Read the model definition and answer for the solid it produces. Units are mm, in the model's axes. Give positions to 0.01 mm unless a question says otherwise; leave off trailing zeros. Order: outer loops, then holes, each group sorted by start corner. A loop starts at its lowest first (then second) coordinate and runs counter-clockwise, first axis right, second up. Notation, with made-up numbers: (-32.75, -18.5) - (19.25, -18.5) arc R18 ccw to (19.25, 15.5) - close; hole circle Ø2 at (-29.75, 6.25). An arc over 180 degrees is marked (long way). Return JSON: item names as keys, results as strings.
```python
from build123d import *

# Parameters (mm, degrees)
SKETCH_1_W               = 40
SKETCH_1_H               = 20
EXTRUDE_2_DEPTH          = 150
SKETCH_5_R               = 20
EXTRUDE_3_DEPTH          = 20
CUT_EXTRUDE_1_DEPTH      = 153.643375225
CUT_EXTRUDE_1_DEPTH_BACK = 153.643375225
SKETCH_6_R               = 10


with BuildPart() as part:
    # 스케치1 → 보스-돌출2 (new body)
    with BuildSketch(Plane.XY):
        Rectangle(SKETCH_1_W, SKETCH_1_H)
    extrude(amount=EXTRUDE_2_DEPTH)

    # 스케치5 → 보스-돌출3 (add)
    with BuildSketch(Plane(origin=(0, 10, 0), x_dir=(1, 0, 0), z_dir=(0, 1, 0))):
        Circle(SKETCH_5_R)
    extrude(amount=-EXTRUDE_3_DEPTH)

    # 스케치6 → 컷-돌출1 (cut, two sides: drawn at the far end of the back side and taken through both)
    with BuildSketch(Plane(origin=(0, 10, 0), x_dir=(1, 0, 0), z_dir=(0, 1, 0)).offset(-CUT_EXTRUDE_1_DEPTH_BACK)):
        with Locations(Location((0, 0, 0), (0, 0, 180))):
            Circle(SKETCH_6_R)
    extrude(amount=CUT_EXTRUDE_1_DEPTH + CUT_EXTRUDE_1_DEPTH_BACK, mode=Mode.SUBTRACT)


solid = part.part
```
Q1. Determine the mould class of faces 1 (the flat face through (-20, 0, 74)), 2 (the cylindrical face through (10, 0, 0)), 3 (the flat face through (20, 0, 74)) for opening direction X: released by +X, released by -X, zero draft, split by the parting line, or undercut.
Values:
{"face 1": "released by -X", "face 2": "undercut", "face 3": "released by +X"}
Q2. A cutting plane is placed at D-D (x = 12). Write down the section's boundary in (y, z).
Values:
{"outline": "(-10, -16) - (10, -16) - (10, 150) - (-10, 150) - close"}
Q3. Consider L1, parallel to Z at x = 0, y = 2.75; L2, parallel to X at y = 3.5, z = 0; L3, parallel to Z at x = -8.5, y = 8.25. Determine where each line is inside the solid, lowest interval first.
Values:
{"L1": "z = -20 to -10, 10 to 150", "L2": "x = -20 to -10, 10 to 20", "L3": "z = -18.1 to -5.27, 5.27 to 150"}
Q4. A cutting plane is placed at C-C (y = 2.25). Write down the section's boundary in (x, z), and give its area (3 significant figures).
Values:
{"outline": "(-20, 0) arc R20 ccw to (20, 0) - (20, 150) - (-20, 150) - close; hole circle Ø20 at (0, 0)", "area": "6,310 mm²"}
Q5. A cutting plane is placed at A-A (x = 0). Write down the section's boundary in (y, z).
Values:
{"outline": "(-10, -20) - (10, -20) - (10, -10) - (-10, -10) - close; (-10, 10) - (10, 10) - (10, 150) - (-10, 150) - close"}
Q6. A cutting plane is placed at B-B (z = -6.5). Write down the section's boundary in (x, y).
Values:
{"outline": "(-18.91, -10) - (-7.6, -10) - (-7.6, 10) - (-18.91, 10) - close; (7.6, -10) - (18.91, -10) - (18.91, 10) - (7.6, 10) - close"}
Q7. Given pin 1 (16 mm diameter, centred on x = 0, z = 0, fed in from +Y); pin 2 (6 mm diameter, centred on x = 10, y = -6.5, fed in from -Z) (3 decimals); pin 3 (3 mm diameter, centred on x = 1, y = -2.5, fed in from -Z), each flat-ended and moving along its own axis, determine where each tip first touches the part or whether it passes through.
Values:
{"pin 1": "passes through", "pin 2": "stops at z = -18.735", "pin 3": "stops at z = -20"}
